Input: part model. Units: mm. Frame: model coordinates. A direction names the side the tool comes from. Coordinates: 2 decimals unless noted, no trailing zeros. Loops run counter-clockwise (first coordinate to the right, second up) from the corner with the lowest first, then second, coordinate; pieces in that order, holes last. Notation, with made-up numbers: (-33.5, 61.25) - (19.5, 61.25) arc R22 cw to (19.5, 76.25) - close; hole circle Ø1 at (-0.5, 77). An arc over 180 degrees is marked (long way). Use a Markdown table: item, result. Add a question column.
1. Section query B-B on x = 0. Return the cut outline in (y, z).
2. Section query A-A on z = -19.25. Return the cut outline in (x, y), then the cut area to 3 significant figures.
3. Ray query, L1, parallel to Y at x = -37, z = -5.5; L2, parallel to Y at x = 0, z = -2.5; L3, parallel to X at y = 11, z = -22. Return the intervals inside material, ascending. Write a range as [from, to].
4. Access query for faces 4 (the face through (-7.255, -42.639, -5.465)), 5 (the face through (45.5, 0, -5)), 6 (the face through (-37, 43.5, -5)). Directions: +Z, -Z, +X, -X, +Y, -Y. A direction counts if a zero-diameter tool reaches every point of the face in a straight line with its end or side. Return the directions, or none.
5. Section query C-C on y = 17.75. Return the cut outline in (x, z) (3 decimals).
6. Contact query for flat-ended pins moving along their axis: P1, Ø1.5, axis at y = -15.5, z = -21.5, coming from the +X side; P2, Ø2, axis at x = -4.5, y = -2.5, coming from the -Z side; P3, Ø2.5, axis at x = 37, y = -39.5, coming from the -Z side; P4, Ø12, axis at y = -28, z = -22, coming from the -X side. Output: stop coordinate, or through.
7. Draft query along Y for faces 1 (the face through (-30, 18, -10)), 2 (the face through (-37, -43.5, -5)), 3 (the face through (41, 40, -5)). Return one class per face: released by +Y, released by -Y, zero draft, split by the parting line, or undercut.
8. Section query D-D on x = 18. Return the cut outline in (y, z).
```python
from build123d import *

# Parameters (mm, degrees)
SKETCH2_W           = 96
SKETCH2_H           = 96
BOSS_EXTRUDE1_DEPTH = 3
BOSS_EXTRUDE2_DEPTH = 27
BOSS_EXTRUDE6_DEPTH = 5
SKETCH18_R          = 1.5
CUT_EXTRUDE3_DEPTH  = 75.215901261
SKETCH16_W          = 5
SKETCH16_H          = 9.5
BOSS_EXTRUDE7_DEPTH = 15
SKETCH17_R          = 1.5
CUT_EXTRUDE2_DEPTH  = 3.175
FILLET2_R           = 1
SKETCH22_R          = 1.5
CUT_EXTRUDE5_DEPTH  = 75.215901261
CUT_EXTRUDE6_START  = -22
SKETCH23_R          = 1.5
CUT_EXTRUDE6_DEPTH  = 22
SKETCH24_W          = 82
SKETCH24_H          = 87
SKETCH24_W_2        = 76
SKETCH24_H_2        = 81
CUT_EXTRUDE8_DEPTH  = 22


with BuildPart() as part:
    # Sketch2 → Boss-Extrude1 (new body)
    with BuildSketch(Plane.XY):
        Rectangle(SKETCH2_W, SKETCH2_H)
    extrude(amount=-BOSS_EXTRUDE1_DEPTH)

    # Sketch3 → Boss-Extrude2 (add)
    with BuildSketch(Plane(origin=(0, 0, -3), x_dir=(-1, 0, 0), z_dir=(0, 0, -1))):
        with BuildLine():
            ThreePointArc((-33, -42.5), (-32.414213562, -41.085786438), (-31, -40.5))
            Line((-31, -40.5), (31, -40.5))
            ThreePointArc((31, -40.5), (32.414213562, -41.085786438), (33, -42.5))
            Line((33, -42.5), (33, -43.5))
            Line((33, -43.5), (41, -43.5))
            Line((41, -43.5), (41, -35.5))
            Line((41, -35.5), (40, -35.5))
            ThreePointArc((40, -35.5), (38.585786438, -34.914213562), (38, -33.5))
            Line((38, -33.5), (38, 33.5))
            ThreePointArc((38, 33.5), (38.585786438, 34.914213562), (40, 35.5))
            Line((40, 35.5), (41, 35.5))
            Line((41, 35.5), (41, 43.5))
            Line((41, 43.5), (33, 43.5))
            Line((33, 43.5), (33, 42.5))
            ThreePointArc((33, 42.5), (32.414213562, 41.085786438), (31, 40.5))
            Line((31, 40.5), (-31, 40.5))
            ThreePointArc((-31, 40.5), (-32.414213562, 41.085786438), (-33, 42.5))
            Line((-33, 42.5), (-33, 43.5))
            Line((-33, 43.5), (-41, 43.5))
            Line((-41, 43.5), (-41, 35.5))
            Line((-41, 35.5), (-40, 35.5))
            ThreePointArc((-40, 35.5), (-38.585786438, 34.914213562), (-38, 33.5))
            Line((-38, 33.5), (-38, -33.5))
            ThreePointArc((-38, -33.5), (-38.585786438, -34.914213562), (-40, -35.5))
            Line((-40, -35.5), (-41, -35.5))
            Line((-41, -35.5), (-41, -43.5))
            Line((-41, -43.5), (-33, -43.5))
            Line((-33, -43.5), (-33, -42.5))
        make_face()
        with BuildLine():
            Line((-35, -22.5), (-35, 22.5))
            ThreePointArc((-35, 22.5), (-30.606601718, 33.106601718), (-20, 37.5))
            Line((-20, 37.5), (20, 37.5))
            ThreePointArc((20, 37.5), (30.606601718, 33.106601718), (35, 22.5))
            Line((35, 22.5), (35, -22.5))
            ThreePointArc((35, -22.5), (30.606601718, -33.106601718), (20, -37.5))
            Line((20, -37.5), (-20, -37.5))
            ThreePointArc((-20, -37.5), (-30.606601718, -33.106601718), (-35, -22.5))
        make_face(mode=Mode.SUBTRACT)
    extrude(amount=BOSS_EXTRUDE2_DEPTH)

    # Sketch15 → Boss-Extrude6 (add)
    with BuildSketch(Plane(origin=(0, 0, -3), x_dir=(-1, 0, 0), z_dir=(0, 0, -1))):
        with BuildLine():
            Line((-5, 48), (5, 48))
            ThreePointArc((5, 48), (7.196699141, 42.696699141), (12.5, 40.5))
            Line((12.5, 40.5), (-12.5, 40.5))
            ThreePointArc((-12.5, 40.5), (-7.196699141, 42.696699141), (-5, 48))
        make_face()
        with BuildLine():
            Line((45.5, 5), (45.5, -5))
            ThreePointArc((45.5, -5), (40.196699141, -7.196699141), (38, -12.5))
            Line((38, -12.5), (38, 12.5))
            ThreePointArc((38, 12.5), (40.196699141, 7.196699141), (45.5, 5))
        make_face()
        with BuildLine():
            Line((5, -48), (-5, -48))
            ThreePointArc((-5, -48), (-7.196699141, -42.696699141), (-12.5, -40.5))
            Line((-12.5, -40.5), (12.5, -40.5))
            ThreePointArc((12.5, -40.5), (7.196699141, -42.696699141), (5, -48))
        make_face()
        with BuildLine():
            Line((-45.5, -5), (-45.5, 5))
            ThreePointArc((-45.5, 5), (-40.196699141, 7.196699141), (-38, 12.5))
            Line((-38, 12.5), (-38, -12.5))
            ThreePointArc((-38, -12.5), (-40.196699141, -7.196699141), (-45.5, -5))
        make_face()
    extrude(amount=BOSS_EXTRUDE6_DEPTH)

    # Sketch18 → Cut-Extrude3 (cut, through all)
    with BuildSketch(Plane.XY):
        with Locations((0, 44.25)):
            Circle(SKETCH18_R)
        with Locations((0, -44.25)):
            Circle(SKETCH18_R)
        with Locations((41.75, 0)):
            Circle(SKETCH18_R)
        with Locations((-41.75, 0)):
            Circle(SKETCH18_R)
    extrude(amount=-CUT_EXTRUDE3_DEPTH, mode=Mode.SUBTRACT)

    # Sketch16 → Boss-Extrude7 (add)
    with BuildSketch(Plane(origin=(0, 0, -3), x_dir=(-1, 0, 0), z_dir=(0, 0, -1))):
        with Locations((-32.5, 17.75)):
            Rectangle(SKETCH16_W, SKETCH16_H)
        with Locations((32.5, 17.75)):
            Rectangle(SKETCH16_W, SKETCH16_H)
    extrude(amount=BOSS_EXTRUDE7_DEPTH)

    # Sketch17 → Cut-Extrude2 (cut)
    with BuildSketch(Plane(origin=(0, 0, -18), x_dir=(-1, 0, 0), z_dir=(0, 0, -1))):
        with Locations((-32.5, 17.75)):
            Circle(SKETCH17_R)
        with Locations((32.5, 17.75)):
            Circle(SKETCH17_R)
    extrude(amount=-CUT_EXTRUDE2_DEPTH, mode=Mode.SUBTRACT)

    # Fillet2
    fillet2_edges = [part.edges().sort_by_distance(p)[0] for p in [
        (-33, 43.5, -16.5),
        (-41, 35.5, -16.5),
        (-41, 43.5, -16.5),
        (33, 43.5, -16.5),
        (41, 43.5, -16.5),
        (41, 35.5, -16.5),
        (41, -35.5, -16.5),
        (33, -43.5, -16.5),
        (-33, -43.5, -16.5),
        (-41, -35.5, -16.5),
        (-41, -43.5, -16.5),
        (41, -43.5, -16.5),
    ]]
    fillet(fillet2_edges, radius=FILLET2_R - 0.0001)  # a hair under: the kernel refuses the full size

    # Sketch22 → Cut-Extrude5 (cut, through all)
    with BuildSketch(Plane.XY):
        with Locations((37, 39.5)):
            Circle(SKETCH22_R)
        with Locations(Location((-37, 39.5, 0), (0, 0, 180))):
            Circle(SKETCH22_R)
        with Locations(Location((37, -39.5, 0), (0, 0, 180))):
            Circle(SKETCH22_R)
        with Locations((-37, -39.5)):
            Circle(SKETCH22_R)
    extrude(amount=-CUT_EXTRUDE5_DEPTH, mode=Mode.SUBTRACT)

    # Sketch23 → Cut-Extrude6 (cut)
    # profile 1 of 4: a face of its own
    with BuildSketch(Plane(origin=(0, 0, -30), x_dir=(-1, 0, 0), z_dir=(0, 0, -1)).offset(CUT_EXTRUDE6_START)):
        with BuildLine():
            ThreePointArc((34, 35.5), (33.292893219, 35.792893219), (33, 36.5))
            Line((33, 36.5), (33, 42.5))
            ThreePointArc((33, 42.5), (33.292893219, 43.207106781), (34, 43.5))
            Line((34, 43.5), (40, 43.5))
            ThreePointArc((40, 43.5), (40.707106781, 43.207106781), (41, 42.5))
            Line((41, 42.5), (41, 36.5))
            ThreePointArc((41, 36.5), (40.707106781, 35.792893219), (40, 35.5))
            Line((40, 35.5), (34, 35.5))
        make_face()
        with Locations(Location((37, 39.5, 0), (0, 0, 180))):
            Circle(SKETCH23_R, mode=Mode.SUBTRACT)
    # profile 2 of 4: a face of its own
    with BuildSketch(Plane(origin=(0, 0, -30), x_dir=(-1, 0, 0), z_dir=(0, 0, -1)).offset(CUT_EXTRUDE6_START)):
        with BuildLine():
            Line((-34, 35.5), (-40, 35.5))
            ThreePointArc((-40, 35.5), (-40.707106781, 35.792893219), (-41, 36.5))
            Line((-41, 36.5), (-41, 42.5))
            ThreePointArc((-41, 42.5), (-40.707106781, 43.207106781), (-40, 43.5))
            Line((-40, 43.5), (-34, 43.5))
            ThreePointArc((-34, 43.5), (-33.292893219, 43.207106781), (-33, 42.5))
            Line((-33, 42.5), (-33, 36.5))
            ThreePointArc((-33, 36.5), (-33.292893219, 35.792893219), (-34, 35.5))
        make_face()
        with Locations(Location((-37, 39.5, 0), (0, 0, 180))):
            Circle(SKETCH23_R, mode=Mode.SUBTRACT)
    # profile 3 of 4: a face of its own
    with BuildSketch(Plane(origin=(0, 0, -30), x_dir=(-1, 0, 0), z_dir=(0, 0, -1)).offset(CUT_EXTRUDE6_START)):
        with BuildLine():
            ThreePointArc((-34, -35.5), (-33.292893219, -35.792893219), (-33, -36.5))
            Line((-33, -36.5), (-33, -42.5))
            ThreePointArc((-33, -42.5), (-33.292893219, -43.207106781), (-34, -43.5))
            Line((-34, -43.5), (-40, -43.5))
            ThreePointArc((-40, -43.5), (-40.707106781, -43.207106781), (-41, -42.5))
            Line((-41, -42.5), (-41, -36.5))
            ThreePointArc((-41, -36.5), (-40.707106781, -35.792893219), (-40, -35.5))
            Line((-40, -35.5), (-34, -35.5))
        make_face()
        with Locations(Location((-37, -39.5, 0), (0, 0, 180))):
            Circle(SKETCH23_R, mode=Mode.SUBTRACT)
    # profile 4 of 4: a face of its own
    with BuildSketch(Plane(origin=(0, 0, -30), x_dir=(-1, 0, 0), z_dir=(0, 0, -1)).offset(CUT_EXTRUDE6_START)):
        with BuildLine():
            Line((34, -35.5), (40, -35.5))
            ThreePointArc((40, -35.5), (40.707106781, -35.792893219), (41, -36.5))
            Line((41, -36.5), (41, -42.5))
            ThreePointArc((41, -42.5), (40.707106781, -43.207106781), (40, -43.5))
            Line((40, -43.5), (34, -43.5))
            ThreePointArc((34, -43.5), (33.292893219, -43.207106781), (33, -42.5))
            Line((33, -42.5), (33, -36.5))
            ThreePointArc((33, -36.5), (33.292893219, -35.792893219), (34, -35.5))
        make_face()
        with Locations(Location((37, -39.5, 0), (0, 0, 180))):
            Circle(SKETCH23_R, mode=Mode.SUBTRACT)
    extrude(amount=CUT_EXTRUDE6_DEPTH, mode=Mode.SUBTRACT)

    # Sketch24 → Cut-Extrude8 (cut)
    with BuildSketch(Plane(origin=(0, 0, -30), x_dir=(-1, 0, 0), z_dir=(0, 0, -1))):
        Rectangle(SKETCH24_W, SKETCH24_H)
        Rectangle(SKETCH24_W_2, SKETCH24_H_2, mode=Mode.SUBTRACT)
    extrude(amount=-CUT_EXTRUDE8_DEPTH, mode=Mode.SUBTRACT)


solid = part.part
```
Resolved:
| question | item | result |
|---|---|---|
| 1 | outline | (-48, -8) - (-45.75, -8) - (-45.75, 0) - (-48, 0) - close; (-42.75, -8) - (-40.5, -8) - (-40.5, -30) - (-37.5, -30) - (-37.5, -3) - (37.5, -3) - (37.5, -30) - (40.5, -30) - (40.5, -8) - (42.75, -8) - (42.75, 0) - (-42.75, 0) - close; (45.75, -8) - (48, -8) - (48, 0) - (45.75, 0) - close |
| 2 | outline | (-38, -35.5) - (-34, -35.5) arc R1 cw to (-33, -36.5) - (-33, -40.5) - (33, -40.5) - (33, -36.5) arc R1 cw to (34, -35.5) - (38, -35.5) - (38, 35.5) - (34, 35.5) arc R1 cw to (33, 36.5) - (33, 40.5) - (-33, 40.5) - (-33, 36.5) arc R1 cw to (-34, 35.5) - (-38, 35.5) - close; hole (-35, -22.5) arc R15 ccw to (-20, -37.5) - (20, -37.5) arc R15 ccw to (35, -22.5) - (35, 22.5) arc R15 ccw to (20, 37.5) - (-20, 37.5) arc R15 ccw to (-35, 22.5) - close |
| 2 | area | 1,000 mm² |
| 3 | L1 | [-43.5, -41], [-38, 38], [41, 43.5] |
| 3 | L2 | [-48, -45.75], [-42.75, 42.75], [45.75, 48] |
| 3 | L3 | [-38, -35], [35, 38] |
| 4 | face 4 | -Z, -Y |
| 4 | face 5 | -Z, +X, +Y, -Y |
| 4 | face 6 | -Z, -X, +Y |
| 5 | outline | (-48, -3) - (-38, -3) - (-38, -30) - (-35, -30) - (-35, -18) - (-34, -18) - (-34, -14.825) - (-31, -14.825) - (-31, -18) - (-30, -18) - (-30, -3) - (30, -3) - (30, -18) - (31, -18) - (31, -14.825) - (34, -14.825) - (34, -18) - (35, -18) - (35, -30) - (38, -30) - (38, -3) - (48, -3) - (48, 0) - (-48, 0) - close |
| 6 | P1 | x = 38 |
| 6 | P2 | z = -3 |
| 6 | P3 | through |
| 6 | P4 | x = -38 |
| 7 | face 1 | undercut |
| 7 | face 2 | released by -Y |
| 7 | face 3 | zero draft |
| 8 | outline | (-48, -3) - (-40.5, -3) - (-40.5, -30) - (-37.5, -30) - (-37.5, -3) - (37.5, -3) - (37.5, -30) - (40.5, -30) - (40.5, -3) - (48, -3) - (48, 0) - (-48, 0) - close |
